Could you check a few things on this model? Use its own coordinates, in mm. A direction names the side the tool comes from. Coordinates: 2 decimals unless noted, no trailing zeros. Order: outer loops, then holes, each group sorted by start corner. A loop starts at its lowest first (then second) coordinate and runs counter-clockwise, first axis right, second up. Notation, with made-up numbers: (32, 41.5) - (63, 41.5) arc R29 ccw to (63, 63.5) - close; hole circle Ø3 at (52, 21). An arc over 180 degrees is marked (long way). One line per item, written item: value.
from build123d import *

# Parameters (mm, degrees)
SKETCH1_R            = 20
SKETCH1_R_2          = 15
BOSS_EXTRUDE1_DEPTH  = 42.5
BOSS_EXTRUDE2_START  = -10
SKETCH2_R            = 30
SKETCH2_R_2          = 20
BOSS_EXTRUDE2_DEPTH  = 10
M4_TAPPED_HOLE1_D    = 3.3
CIRPATTERN1_COUNT    = 6
SKETCH5_R            = 21.5
SKETCH5_R_2          = 19
CUT_EXTRUDE1_DEPTH   = 1.4
FILLET1_R            = 0.5
MIRROR1_COPY_1_D     = 3.3
MIRROR1_COPY_2_D     = 3.3
MIRROR1_COPY_3_D     = 3.3
MIRROR1_COPY_4_D     = 3.3
MIRROR1_COPY_5_D     = 3.3
FILLET1_OF_MIRROR1_R = 0.5


with BuildPart() as part:
    # Sketch1 → Boss-Extrude1 (new, symmetric)
    with BuildSketch(Plane.XY):
        Circle(SKETCH1_R)
        Circle(SKETCH1_R_2, mode=Mode.SUBTRACT)
    extrude(amount=BOSS_EXTRUDE1_DEPTH, both=True)

    # Sketch2 → Boss-Extrude2 (add)
    with BuildSketch(Plane(origin=(0, 0, -42.5), x_dir=(-1, 0, 0), z_dir=(0, 0, -1)).offset(BOSS_EXTRUDE2_START)):
        Circle(SKETCH2_R)
        Circle(SKETCH2_R_2, mode=Mode.SUBTRACT)
    boss_extrude2 = extrude(amount=BOSS_EXTRUDE2_DEPTH)

    # M4 Tapped Hole1 (through all)
    with Locations(Plane(origin=(0, 0, -42.5), x_dir=(-1, 0, 0), z_dir=(0, 0, -1))):
        with Locations((0, 24.5)):
            m4_tapped_hole1 = Hole(M4_TAPPED_HOLE1_D / 2)

    # CirPattern1: M4 Tapped Hole1 ×6 about axis
    cirpattern1_axis = Axis((0, 0, 0), (0, 0, 1))
    for i in range(1, CIRPATTERN1_COUNT):
        add(m4_tapped_hole1.rotate(cirpattern1_axis, i * 360 / CIRPATTERN1_COUNT), mode=Mode.SUBTRACT)

    # Sketch5 → Cut-Extrude1 (cut)
    with BuildSketch(Plane(origin=(0, 0, -42.5), x_dir=(-1, 0, 0), z_dir=(0, 0, -1))):
        Circle(SKETCH5_R)
        Circle(SKETCH5_R_2, mode=Mode.SUBTRACT)
    cut_extrude1 = extrude(amount=-CUT_EXTRUDE1_DEPTH, mode=Mode.SUBTRACT)

    # Fillet1
    fillet1_edges = [part.edges().sort_by_distance(p)[0] for p in [
        (21.5, 0, -41.1),
        (19, 0, -41.1),
    ]]
    fillet(fillet1_edges, radius=FILLET1_R)

    # Mirror1: Boss-Extrude2, M4 Tapped Hole1, Cut-Extrude1 across plane
    add(boss_extrude2.mirror(Plane.XY))
    add(m4_tapped_hole1.mirror(Plane.XY), mode=Mode.SUBTRACT)
    add(cut_extrude1.mirror(Plane.XY), mode=Mode.SUBTRACT)

    # Mirror1 copy 1 (through all)
    with Locations(Plane(origin=(0, 0, 42.5), x_dir=(-0.5000000000000001, -0.8660254037844386, 0), z_dir=(0, 0, 1))):
        with Locations((0, -24.5)):
            Hole(MIRROR1_COPY_1_D / 2)

    # Mirror1 copy 2 (through all)
    with Locations(Plane(origin=(0, 0, 42.5), x_dir=(0.4999999999999998, -0.8660254037844387, 0), z_dir=(0, 0, 1))):
        with Locations((0, -24.5)):
            Hole(MIRROR1_COPY_2_D / 2)

    # Mirror1 copy 3 (through all)
    with Locations(Plane.XY.offset(42.5)):
        with Locations((0, -24.5)):
            Hole(MIRROR1_COPY_3_D / 2)

    # Mirror1 copy 4 (through all)
    with Locations(Plane(origin=(0, 0, 42.5), x_dir=(0.5000000000000004, 0.8660254037844384, 0), z_dir=(0, 0, 1))):
        with Locations((0, -24.5)):
            Hole(MIRROR1_COPY_4_D / 2)

    # Mirror1 copy 5 (through all)
    with Locations(Plane(origin=(0, 0, 42.5), x_dir=(-0.5000000000000001, 0.8660254037844386, 0), z_dir=(0, 0, 1))):
        with Locations((0, -24.5)):
            Hole(MIRROR1_COPY_5_D / 2)

    # Fillet1 of Mirror1
    fillet1_of_mirror1_edges = [part.edges().sort_by_distance(p)[0] for p in [
        (21.5, 0, 41.1),
        (19, 0, 41.1),
    ]]
    fillet(fillet1_of_mirror1_edges, radius=FILLET1_OF_MIRROR1_R)


solid = part.part
Item 1: I want a section at C-C on z = -20. Please give me the cut outline in (x, y).
Conclusion:
outline: circle Ø40 at (0, 0); hole circle Ø30 at (0, 0)
Item 2: Thinking about a two-plate mould opening in Y: for faces 1 (the face through (0.215, -22.864, 37.43)), 2 (the face through (29.97, 1.32, 37.43)), 3 (the face through (-9, -20, 42.5)), 4 (the face through (-8.767, -16.856, 42.056)), which applies, pulls with the +Y half, pulls with the -Y half, needs draft (parallel to the pull), parting line crosses it, or undercut?
Conclusion:
face 1: undercut
face 2: parting line crosses it
face 3: needs draft
face 4: undercut
Item 3: I want a section at A-A on y = -24.5. Please give me the cut outline in (x, z).
Conclusion:
outline: (-17.31, -42.5) - (-1.65, -42.5) - (-1.65, -32.5) - (-17.31, -32.5) - close; (-17.31, 32.5) - (-1.65, 32.5) - (-1.65, 42.5) - (-17.31, 42.5) - close; (1.65, -42.5) - (17.31, -42.5) - (17.31, -32.5) - (1.65, -32.5) - close; (1.65, 32.5) - (17.31, 32.5) - (17.31, 42.5) - (1.65, 42.5) - close
Item 4: For faces 5 (the face through (-4.336, -19.524, 0.455)), 6 (the face through (-6, -19, 41.1)), 7 (the face through (-19.908, 13.254, -37.43)), which set-ups out of +Z, -Z, +X, -X, +Y, -Y let a thin tool reach every point of the face, with its end or its side?
Conclusion:
face 5: none
face 6: +Z
face 7: +Z, -Z
Item 5: If I drill on probe 1 along Y at (x, z) = (0, -15); probe 2 along Z at (x, y) = (7, 22.5); probe 3 along Z at (x, y) = (12.5, -16), over which ranges is the centre line in solid material (lowest first)?
Conclusion:
probe 1: -20 to -15, 15 to 20
probe 2: -42.5 to -32.5, 32.5 to 42.5
probe 3: -41.1 to -32.5, 32.5 to 41.1
Item 6: I'm going to push flat-ended pins straight in: pin 1 Ø2.5 at (x, y) = (-21.22, -12.25) entering from +Z; pin 2 Ø5.5 at (x, y) = (21.22, -12.25) entering from +Z; pin 3 Ø10 at (x, z) = (11.5, -5) entering from +Y; pin 4 Ø1.5 at (x, z) = (-10, 7) entering from -Y. Where does each tip first touch, or does it pass through?
Conclusion:
pin 1: through
pin 2: z = 42.5
pin 3: y = 18.91
pin 4: y = -17.73
Item 7: I want a section at B-B on x = 0. Give the number of separate pieces and of enclosed holes in the cut face, then the cut area to 3 significant figures.
Conclusion:
separate pieces: 6
enclosed holes: 0
area: 1,100 mm²
